```python
from build123d import *

# Parameters (mm, degrees)
SKETCH1_W           = 46
SKETCH1_H           = 20
BOSS_EXTRUDE1_DEPTH = 1
SKETCH2_R           = 8
SKETCH2_R_2         = 6
BOSS_EXTRUDE2_DEPTH = 12
SKETCH3_W           = 5.881600094
SKETCH3_H           = 1.447060341
BOSS_EXTRUDE3_DEPTH = 5


with BuildPart() as part:
    # Sketch1 → Boss-Extrude1 (new body, symmetric)
    with BuildSketch(Plane(origin=(0, 0, 0), x_dir=(0, 0, -1), z_dir=(1, 0, 0))):
        with Locations((23, 10)):
            Rectangle(SKETCH1_W, SKETCH1_H)
    extrude(amount=BOSS_EXTRUDE1_DEPTH, both=True)

    # Sketch2 → Boss-Extrude2 (add)
    with BuildSketch(Plane(origin=(1, 0, 0), x_dir=(0, 0, -1), z_dir=(1, 0, 0))):
        with Locations((9, 10)):
            Circle(SKETCH2_R)
        with Locations((9, 10)):
            Circle(SKETCH2_R_2, mode=Mode.SUBTRACT)
        with Locations((37, 10)):
            Circle(SKETCH2_R)
        with Locations((37, 10)):
            Circle(SKETCH2_R_2, mode=Mode.SUBTRACT)
    extrude(amount=BOSS_EXTRUDE2_DEPTH)

    # Sketch3 → Boss-Extrude3 (add)
    with BuildSketch(Plane.ZY.offset(1)):
        with Locations((-22.486526976, 0.723530171)):
            Rectangle(SKETCH3_W, SKETCH3_H)
    extrude(amount=BOSS_EXTRUDE3_DEPTH)


solid = part.part
```
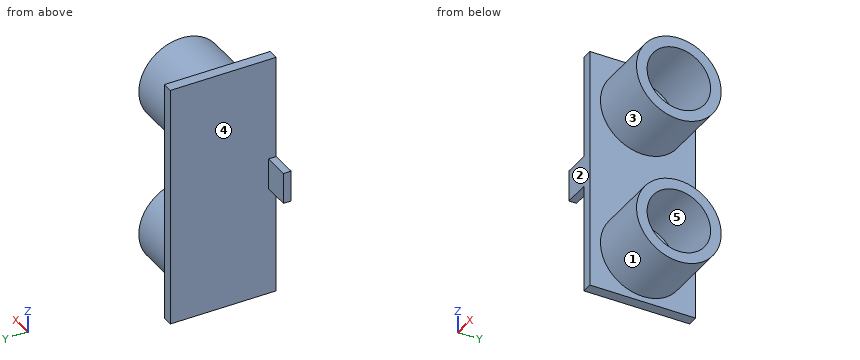
Here's how the part is built. I have some questions about the finished solid (model axes, mm). Face numbers are marked on the shaded views. A direction names the side the tool comes from. Round coordinates to 2 decimals unless told otherwise and drop trailing zeros. Loops run counter-clockwise (first coordinate to the right, second up) from the corner with the lowest first, then second, coordinate; pieces in that order, holes last.
1. Will these pins go through, and if not, where does the flat tip stop? pin 1 (1.5 mm diameter, centred on x = -3.5, z = -21, fed in from +Y); pin 2 (1.2 mm diameter, centred on x = -4, y = 1, fed in from +Z); pin 3 (10 mm diameter, centred on x = 9, y = 11.5, fed in from -Z).
Answers:
pin 1: stops at y = 1.45
pin 2: stops at z = -19.55
pin 3: stops at z = -45
2. Suppose I cut it at C-C, the plane z = -9. Please give me the cut outline in (x, y), and give its area (3 significant figures).
Answers:
outline: (-1, 0) - (1, 0) - (1, 2) - (13, 2) - (13, 4) - (1, 4) - (1, 16) - (13, 16) - (13, 18) - (1, 18) - (1, 20) - (-1, 20) - close
area: 88.0 mm2
3. For the marked faces 1 and 2, which set-ups out of +Z, -Z, +X, -X, +Y, -Y let a thin tool reach every point of the face, with its end or its side?
Answers:
face 1: +X
face 2: +Z, -Z, +X, -X, -Y
4. Suppose I cut it at D-D, the plane x = -3.75. Please give me the cut outline in (y, z).
Answers:
outline: (0, -25.43) - (1.45, -25.43) - (1.45, -19.55) - (0, -19.55) - close
5. Suppose I cut it at A-A, the plane x = 11.25. Please give me the cut outline in (y, z).
Answers:
outline: circle Ø16 at (10, -37); circle Ø16 at (10, -9); hole circle Ø12 at (10, -37); hole circle Ø12 at (10, -9)
6. Suppose I cut it at B-B, the plane y = 10. Please give me the cut outline in (x, z).
Answers:
outline: (-1, -46) - (1, -46) - (1, -45) - (13, -45) - (13, -43) - (1, -43) - (1, -31) - (13, -31) - (13, -29) - (1, -29) - (1, -17) - (13, -17) - (13, -15) - (1, -15) - (1, -3) - (13, -3) - (13, -1) - (1, -1) - (1, 0) - (-1, 0) - close
7. If I drill on probe 1 along Y at (x, z) = (6.75, -9); probe 2 along Z at (x, y) = (7, 6); probe 3 along Z at (x, y) = (11.75, 13.75), over which ranges is the centre line in solid material (lowest first)?
Answers:
probe 1: y = 2 to 4, 16 to 18
probe 2: z = -43.93 to -41.47, -32.53 to -30.07, -15.93 to -13.47, -4.53 to -2.07
probe 3: z = -44.07 to -41.68, -32.32 to -29.93, -16.07 to -13.68, -4.32 to -1.93
8. Thinking about a two-plate mould opening in Y: for the marked faces 3, 4 and 5, which applies, released by +Y, released by -Y, zero draft, split by the parting line, or undercut?
Answers:
face 3: split by the parting line
face 4: zero draft
face 5: undercut
